```python
from build123d import *

# Parameters (mm, degrees)
SKETCH_2_W          = 15
SKETCH_2_H          = 15
SKETCH_2_W_2        = 13
SKETCH_2_H_2        = 13
EXTRUDE_1_DEPTH     = 630
SKETCH_3_R          = 1.6
CUT_EXTRUDE_1_DEPTH = 631.223174756
SKETCH_4_R          = 1.6
CUT_EXTRUDE_2_DEPTH = 631.223174756


with BuildPart() as part:
    # 草图2 → 拉伸-薄壁1 (new body)
    with BuildSketch(Plane(origin=(0, 0, 0), x_dir=(1, 0, 0), z_dir=(0, 1, 0))):
        Rectangle(SKETCH_2_W, SKETCH_2_H)
        Rectangle(SKETCH_2_W_2, SKETCH_2_H_2, mode=Mode.SUBTRACT)
    extrude(amount=EXTRUDE_1_DEPTH)

    # 草图3 → 切除-拉伸1 (cut, through all)
    with BuildSketch(Plane.XY.offset(7.5)):
        with Locations((0, 7.5)):
            Circle(SKETCH_3_R)
        with Locations((0, 22.5)):
            Circle(SKETCH_3_R)
        with Locations((0, 42.5)):
            Circle(SKETCH_3_R)
        with Locations((0, 72.5)):
            Circle(SKETCH_3_R)
        with Locations((0, 315)):
            Circle(SKETCH_3_R)
        with Locations((0, 295)):
            Circle(SKETCH_3_R)
        with Locations((0, 335)):
            Circle(SKETCH_3_R)
        with Locations(Location((0, 557.5, 0), (0, 0, 180))):
            Circle(SKETCH_3_R)
        with Locations(Location((0, 587.5, 0), (0, 0, 180))):
            Circle(SKETCH_3_R)
        with Locations(Location((0, 607.5, 0), (0, 0, 180))):
            Circle(SKETCH_3_R)
        with Locations(Location((0, 622.5, 0), (0, 0, 180))):
            Circle(SKETCH_3_R)
    extrude(amount=-CUT_EXTRUDE_1_DEPTH, mode=Mode.SUBTRACT)

    # 草图4 → 切除-拉伸2 (cut, through all)
    with BuildSketch(Plane(origin=(7.5, 0, 0), x_dir=(0, 0, -1), z_dir=(1, 0, 0))):
        with Locations((0, 290)):
            Circle(SKETCH_4_R)
        with Locations((0, 340)):
            Circle(SKETCH_4_R)
    extrude(amount=-CUT_EXTRUDE_2_DEPTH, mode=Mode.SUBTRACT)


solid = part.part
```
CAD build for the part. Positions are in the model's coordinates, mm. A direction names the side the tool comes from. Round coordinates to 2 decimals unless told otherwise and drop trailing zeros. Write each loop counter-clockwise with the first axis right and the second up, starting at its lowest first coordinate (ties: lowest second). Pieces come first, ordered by that corner, then holes. Notation, with made-up numbers: (32, -14) - (88, -14) arc R13 ccw to (88, -9) - close; hole circle Ø7 at (50, -23). An arc over 180 degrees is marked (long way). Write item = value, one per line. Start each with the question number.
Q1. Probe L1, parallel to Y at x = 7, z = 0; L2, parallel to Z at x = -3.75, y = 420. List the from-to ranges inside material, lowest first. Write a range as from..to.
Q2. Mould opens along X. For faces 1 (the flat face through (7.5, 311, 0)), 2 (the flat face through (6.5, 311, 0)), 3 (the flat face through (-7, 630, 0)) say: pulls with the +X half, pulls with the -X half, needs draft (parallel to the pull), parting line crosses it, or undercut.
Q3. Band-saw the part on A-A (y = 452.5). Give the cut face in (x, z).
Q4. Which spindle directions (+Z, -Z, +X, -X, +Y, -Y) get a long thin tool onto all of the face, cutting with end or side? Do faces 4 (the flat face through (-6.5, 311, 0)), 5 (the flat face through (-7, 0, 0)). Say none if no direction does.
Q5. Drop flat-ended pins along their axis: pin 1 (4 mm diameter, centred on x = 0, y = 22.5, fed in from +Z); pin 2 (5 mm diameter, centred on x = 2.5, z = -3, fed in from +Y). Give the stop position or say it passes through.
Answers below:
q1.L1 = 0..288.4, 291.6..338.4, 341.6..630
q1.L2 = -7.5..-6.5, 6.5..7.5
q2.face_1 = pulls with the +X half
q2.face_2 = undercut
q2.face_3 = needs draft
q3.outline = (-7.5, -7.5) - (7.5, -7.5) - (7.5, 7.5) - (-7.5, 7.5) - close; hole (-6.5, -6.5) - (6.5, -6.5) - (6.5, 6.5) - (-6.5, 6.5) - close
q4.face_4 = +Y, -Y
q4.face_5 = +Z, -Z, +X, -X, -Y
q5.pin_1 = 7.5
q5.pin_2 = through
